from build123d import *

# Parameters (mm, degrees)
BOSS_EXTRUDE1_DEPTH = 4.699
CAVITY1_START       = 10.583333333
CAVITY1_OUTLINE_W   = 4.699
CAVITY1_OUTLINE_H   = 4.699
CAVITY1_DEPTH       = 10.583333334


# Read off the part's stored shape, not the designer's step: Cavity1
with BuildPart() as part:
    # Sketch1 → Boss-Extrude1 (new body)
    with BuildSketch(Plane.XY):
        Polygon((67.733333333, 31.75), (101.6, 31.75), (101.6, 0), (67.733333333, 0), (67.733333333, -4.699), (33.866666667, -4.699), (33.866666667, 0), (0, 0), (0, 31.75), (33.866666667, 31.75), (33.866666667, 36.449), (67.733333333, 36.449), align=None)
    extrude(amount=BOSS_EXTRUDE1_DEPTH)

    # Cavity1 outline → Cavity1 (cut)
    with BuildSketch(Plane(origin=(0, 0, 0), x_dir=(1, 0, 0), z_dir=(0, 1, 0)).offset(CAVITY1_START)):
        with Locations((2.3495, -2.3495)):
            Rectangle(CAVITY1_OUTLINE_W, CAVITY1_OUTLINE_H)
        with Locations((99.2505, -2.3495)):
            Rectangle(CAVITY1_OUTLINE_W, CAVITY1_OUTLINE_H)
    extrude(amount=CAVITY1_DEPTH, mode=Mode.SUBTRACT)


solid = part.part
Can you work these out from the model? Positions are in its coordinate system, mm. A direction names the side the tool comes from. Coordinates: 2 decimals unless noted, no trailing zeros. Order: outer loops, then holes, each group sorted by start corner. A loop starts at its lowest first (then second) coordinate and runs counter-clockwise, first axis right, second up. Notation, with made-up numbers: M 39,-12.5 L 85,-12.5 A21 cw 85,18.5 Z; hole C 51,45.25 d10. An arc over 180 degrees is marked long. Write item = value, one per line.
(1) For faces 1 (the face through (17, 0, 2)), 2 (the face through (85, 0, 2)), 3 (the face through (99, 10.583, 2)), 4 (the face through (33.867, 34, 2)), 5 (the face through (4.699, 16, 2)), which set-ups out of +Z, -Z, +X, -X, +Y, -Y let a thin tool reach every point of the face, with its end or its side?
Results are:
face_1 = +Z, -Z, -X, -Y
face_2 = +Z, -Z, +X, -Y
face_3 = +Z, -Z, +X
face_4 = +Z, -Z, -X, +Y
face_5 = +Z, -Z, -X
(2) Suppose I cut it at B-B on y = 16.5. Please give me the cut outline in (x, z), plus the area to 3 significant figures.
Results are:
outline = M 4.7,0 L 96.9,0 L 96.9,4.7 L 4.7,4.7 Z
area = 433 mm2
(3) Suppose I cut it at C-C on x = 29.5. Please give me the cut outline in (y, z).
Results are:
outline = M 0,0 L 31.75,0 L 31.75,4.7 L 0,4.7 Z
(4) For pin 1 Ø1.4 at (y, z) = (17.5, 1.5) entering from -X; pin 2 Ø1.4 at (x, z) = (17, 2) entering from -Y; pin 3 Ø2.5 at (y, z) = (16.5, 3) entering from +X; pin 4 Ø1 at (y, z) = (6, 3.5) entering from -X, each with a flat end and sliding along its axis, tell me the tip position at first contact or that it passes through.
Results are:
pin_1 = 4.7
pin_2 = 0
pin_3 = 96.9
pin_4 = 0
(5) I need wall thicknesses on line 1 along X through (y, z) = (34.5, 0.6); line 2 along X through (y, z) = (13.5, 2.55); line 3 along Y through (x, z) = (84.5, 1.1). Which ranges of each line are inside material? Lowest first, please. Write a range as [from, to].
Results are:
line_1 = [33.87, 67.73]
line_2 = [4.7, 96.9]
line_3 = [0, 31.75]
(6) If we mould it in two halves opening along Y, with no side actions, what happens to faces 6 (the face through (2, 10.583, 2)), 7 (the face through (84, 31.75, 2)), 8 (the face through (67.733, 34, 2)), 9 (the face through (51, -4.699, 2))? For each: pulls with the +Y half, pulls with the -Y half, needs draft (parallel to the pull), parting line crosses it, or undercut.
Results are:
face_6 = undercut
face_7 = pulls with the +Y half
face_8 = needs draft
face_9 = pulls with the -Y half
(7) Suppose I cut it at A-A on z = 3.95. Please give me the cut outline in (x, y), plus the area to 3 significant figures.
Results are:
outline = M 0,0 L 33.87,0 L 33.87,-4.7 L 67.73,-4.7 L 67.73,0 L 101.6,0 L 101.6,10.58 L 96.9,10.58 L 96.9,21.17 L 101.6,21.17 L 101.6,31.75 L 67.73,31.75 L 67.73,36.45 L 33.87,36.45 L 33.87,31.75 L 0,31.75 L 0,21.17 L 4.7,21.17 L 4.7,10.58 L 0,10.58 Z
area = 3,440 mm2
